```python
from build123d import *
from build123d import SkipClean  # not in build123d's __all__

# Parameters (mm, degrees)
F0_R     = 12.7
F1_DEPTH = 276.86
F3_DEPTH = 2.54
F4_DEPTH = 25.4


with BuildPart() as f1:
    # F0 (on Right) → F1 (new body)
    with BuildSketch(Plane.YZ):
        Circle(F0_R)
    extrude(amount=F1_DEPTH)

    # F2 (on face) → F3 (join)
    with BuildSketch(Plane.YZ.offset(276.86)):
        with BuildLine():
            ThreePointArc((2.54, 5.8198711326), (4.4901280605, 4.4901280605), (5.8198711326, 2.54))
            Line((5.8198711326, 2.54), (12.4434078933, 2.54))
            ThreePointArc((12.4434078933, 2.54), (8.9802561211, 8.9802561211), (2.54, 12.4434078933))
            Line((2.54, 12.4434078933), (2.54, 5.8198711326))
        make_face()
        with BuildLine():
            ThreePointArc((-5.8198711326, 2.54), (-4.4901280605, 4.4901280605), (-2.54, 5.8198711326))
            Line((-2.54, 5.8198711326), (-2.54, 12.4434078933))
            ThreePointArc((-2.54, 12.4434078933), (-8.9802561211, 8.9802561211), (-12.4434078933, 2.54))
            Line((-12.4434078933, 2.54), (-5.8198711326, 2.54))
        make_face()
        with BuildLine():
            Line((-2.54, -12.4434078933), (-2.54, -5.8198711326))
            ThreePointArc((-2.54, -5.8198711326), (-4.4901280605, -4.4901280605), (-5.8198711326, -2.54))
            Line((-5.8198711326, -2.54), (-12.4434078933, -2.54))
            ThreePointArc((-12.4434078933, -2.54), (-8.9802561211, -8.9802561211), (-2.54, -12.4434078933))
        make_face()
        with BuildLine():
            Line((12.4434078933, -2.54), (5.8198711326, -2.54))
            ThreePointArc((5.8198711326, -2.54), (4.4901280605, -4.4901280605), (2.54, -5.8198711326))
            Line((2.54, -5.8198711326), (2.54, -12.4434078933))
            ThreePointArc((2.54, -12.4434078933), (8.9802561211, -8.9802561211), (12.4434078933, -2.54))
        make_face()
    extrude(amount=F3_DEPTH)

    # F2 (on face) → F4 (cut)
    with BuildSketch(Plane.YZ.offset(276.86)):
        with BuildLine():
            ThreePointArc((5.8198711326, -2.54), (6.2160550871, -1.2973662374), (6.35, 0))
            ThreePointArc((6.35, 0), (6.2160550871, 1.2973662374), (5.8198711326, 2.54))
            ThreePointArc((5.8198711326, 2.54), (4.4901280605, 4.4901280605), (2.54, 5.8198711326))
            ThreePointArc((2.54, 5.8198711326), (0, 6.35), (-2.54, 5.8198711326))
            ThreePointArc((-2.54, 5.8198711326), (-4.4901280605, 4.4901280605), (-5.8198711326, 2.54))
            ThreePointArc((-5.8198711326, 2.54), (-6.35, 0), (-5.8198711326, -2.54))
            ThreePointArc((-5.8198711326, -2.54), (-4.4901280605, -4.4901280605), (-2.54, -5.8198711326))
            ThreePointArc((-2.54, -5.8198711326), (0, -6.35), (2.54, -5.8198711326))
            ThreePointArc((2.54, -5.8198711326), (4.4901280605, -4.4901280605), (5.8198711326, -2.54))
        make_face()
    with SkipClean():  # cleaning this boolean's faces spoils the solid; the shape is the same uncleaned
        extrude(amount=-F4_DEPTH, mode=Mode.SUBTRACT)


solid = f1.part
```
Here's how the part is built. I have some questions about the finished solid (model axes, mm). A direction names the side the tool comes from. Give positions to 0.01 mm unless a question says otherwise; leave off trailing zeros. Loops run counter-clockwise (first coordinate to the right, second up) from the corner with the lowest first, then second, coordinate; pieces in that order, holes last. Notation, with made-up numbers: M 35,68 L 70,68 A22 cw 70,102 Z; hole C -19,-11 d3. An arc over 180 degrees is marked long. Return JSON: item names as keys, results as strings.
Item 1: Thinking about a two-plate mould opening in Y: for faces 4 (the flat face through (276.86, 9, 0)), 5 (the flat face through (276.86, 0, 9)), which applies, released by +Y, released by -Y, zero draft, split by the parting line, or undercut?
A:
{"face 4": "zero draft", "face 5": "undercut"}
Item 2: Imagine slicing it at B-B on x = 30. List the corners of the cut face in (y, z) for me.
A:
{"outline": "C 0,0 d25.4"}
Item 3: Imagine slicing it at A-A on y = 0. List the corners of the cut face in (x, z) for me, then the cut area to 3 significant figures.
A:
{"outline": "M 0,-12.7 L 276.86,-12.7 L 276.86,-6.35 L 251.46,-6.35 L 251.46,6.35 L 276.86,6.35 L 276.86,12.7 L 0,12.7 Z", "area": "6,710 mm^2"}
Item 4: On a 3-axis mill with a long thin cutter (end or side, diameter ignored), from which of +Z, -Z, +X, -X, +Y, -Y can I reach the whole of each face in a straight line? I mean faces 1 (the flat face through (251.46, 0, 0)), 2 (the flat face through (276.86, 0, -9)), 3 (the flat face through (276.86, -9, 0)). Say none if no direction works.
A:
{"face 1": "+X", "face 2": "+Z, -Z, +X", "face 3": "+X, +Y, -Y"}
Item 5: Please list where these lines run through material, in increasing order: line 1 (X direction, y = -1.25, z = 6.75); line 2 (Y direction, x = 88.5, z = 2.5); line 3 (Y direction, x = 168.5, z = 0.25).
A:
{"line 1": "x = 0 to 276.86", "line 2": "y = -12.45 to 12.45", "line 3": "y = -12.7 to 12.7"}
Item 6: I'm going to push flat-ended pins straight in: pin 1 Ø1.3 at (x, y) = (278, -8.5) entering from +Z; pin 2 Ø2.5 at (y, z) = (-1, 9.5) entering from +X; pin 3 Ø2 at (x, z) = (278, 8) entering from -Y. Where does each tip first touch, or does it pass through?
A:
{"pin 1": "stops at z = 9.98", "pin 2": "stops at x = 276.86", "pin 3": "stops at y = -10.6"}
